The model under review builds one solid part; all positions refer to its coordinate system, in mm. Coordinates: 2 decimals unless noted, no trailing zeros. Order: outer loops, then holes, each group sorted by start corner. A loop starts at its lowest first (then second) coordinate and runs counter-clockwise, first axis right, second up. Notation, with made-up numbers: (17, 54.25) - (67, 54.25) arc R20 ccw to (67, 77.25) - close; hole circle Ø7 at (64.5, 70). An arc over 180 degrees is marked (long way). Answer in a Markdown table with one row per item.
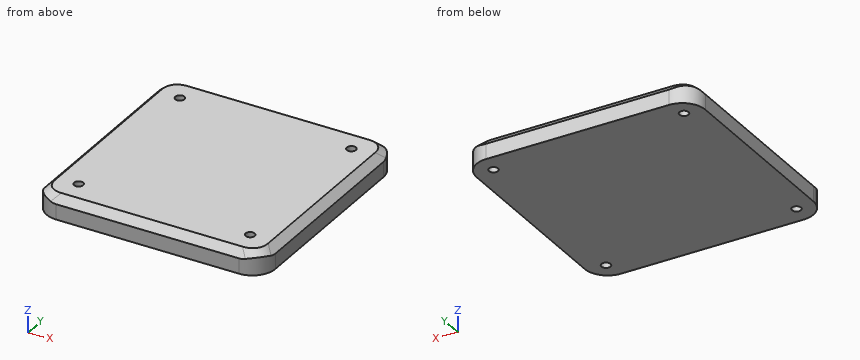
```python
from build123d import *

# Parameters (mm, degrees)
F0_W     = 300
F0_H     = 300
F0_R     = 6
F1_DEPTH = 30
F2_DEPTH = 10
F3_DEPTH = 20
F4_SIZE2 = 10
F4_SIZE  = 10
F5_F1_R  = 30
F5_F2_R  = 30
F5_F3_R  = 30
F5_F4_R  = 30
F5_F5_R  = 30
F5_F6_R  = 30
F5_F7_R  = 30
F5_F8_R  = 30


with BuildPart() as f1:
    # F0 (on Top) → F1 (new body)
    with BuildSketch(Plane.XY):
        Rectangle(F0_W, F0_H)
        with Locations((-125, -125)):
            Circle(F0_R, mode=Mode.SUBTRACT)
        with Locations((-112.5, -112.5)):
            Circle(F0_R, mode=Mode.SUBTRACT)
        with Locations((125, -125)):
            Circle(F0_R, mode=Mode.SUBTRACT)
        with Locations((112.5, -112.5)):
            Circle(F0_R, mode=Mode.SUBTRACT)
        with Locations((-125, 125)):
            Circle(F0_R, mode=Mode.SUBTRACT)
        with Locations((-112.5, 112.5)):
            Circle(F0_R, mode=Mode.SUBTRACT)
        with Locations((112.5, 112.5)):
            Circle(F0_R, mode=Mode.SUBTRACT)
        with Locations((125, 125)):
            Circle(F0_R, mode=Mode.SUBTRACT)
        with Locations((-125, -125)):
            Circle(F0_R)
        with Locations((-125, 125)):
            Circle(F0_R)
        with Locations((125, 125)):
            Circle(F0_R)
        with Locations((125, -125)):
            Circle(F0_R)
    extrude(amount=F1_DEPTH)

    # F0 (on Top) → F2 (cut)
    with BuildSketch(Plane.XY):
        with Locations((-125, -125)):
            Circle(F0_R)
        with Locations((-125, 125)):
            Circle(F0_R)
        with Locations((125, 125)):
            Circle(F0_R)
        with Locations((125, -125)):
            Circle(F0_R)
    extrude(amount=F2_DEPTH, mode=Mode.SUBTRACT)

    # F0 (on Top) → F3 (join)
    with BuildSketch(Plane.XY):
        with Locations((-112.5, 112.5)):
            Circle(F0_R)
        with Locations((-112.5, -112.5)):
            Circle(F0_R)
        with Locations((112.5, 112.5)):
            Circle(F0_R)
        with Locations((112.5, -112.5)):
            Circle(F0_R)
    extrude(amount=F3_DEPTH)

    # F4
    f4_edges = [f1.edges().sort_by_distance(p)[0] for p in [
        (0, -150, 30),
        (-150, 0, 30),
        (150, 0, 30),
        (0, 150, 30),
    ]]
    chamfer(f4_edges, length=F4_SIZE, length2=F4_SIZE2)

    # F5: fillet of radius 30 on 8 edges, made by hand

    # F5_f1
    f5_f1_edges = [f1.edges().sort_by_distance(p)[0] for p in [
        (-150, -150, 10),
    ]]
    fillet(f5_f1_edges, radius=F5_F1_R)

    # F5_f2
    f5_f2_edges = [f1.edges().sort_by_distance(p)[0] for p in [
        (150, -150, 10),
    ]]
    fillet(f5_f2_edges, radius=F5_F2_R)

    # F5_f3
    f5_f3_edges = [f1.edges().sort_by_distance(p)[0] for p in [
        (-150, 150, 10),
    ]]
    fillet(f5_f3_edges, radius=F5_F3_R)

    # F5_f4
    f5_f4_edges = [f1.edges().sort_by_distance(p)[0] for p in [
        (-140.6066017178, -140.6066017178, 29.3933982822),
    ]]
    fillet(f5_f4_edges, radius=F5_F4_R)

    # F5_f5
    f5_f5_edges = [f1.edges().sort_by_distance(p)[0] for p in [
        (140.6066017178, -140.6066017178, 29.3933982822),
    ]]
    fillet(f5_f5_edges, radius=F5_F5_R)

    # F5_f6
    f5_f6_edges = [f1.edges().sort_by_distance(p)[0] for p in [
        (150, 150, 10),
    ]]
    fillet(f5_f6_edges, radius=F5_F6_R)

    # F5_f7
    f5_f7_edges = [f1.edges().sort_by_distance(p)[0] for p in [
        (-140.6066017178, 140.6066017178, 29.3933982822),
    ]]
    fillet(f5_f7_edges, radius=F5_F7_R)

    # F5_f8
    f5_f8_edges = [f1.edges().sort_by_distance(p)[0] for p in [
        (140.6066017178, 140.6066017178, 29.3933982822),
    ]]
    fillet(f5_f8_edges, radius=F5_F8_R)


solid = f1.part
```
Item 1: We need section A-A, the plane y = -112.5. Write out the cut boundary in (x, z).
Check values:
| item | result |
|---|---|
| outline | (-150, 0) - (150, 0) - (150, 20) - (140, 30) - (118.5, 30) - (118.5, 20) - (106.5, 20) - (106.5, 30) - (-106.5, 30) - (-106.5, 20) - (-118.5, 20) - (-118.5, 30) - (-140, 30) - (-150, 20) - close |
Item 2: To check wall thickness, follow line 1 (Y direction, x = 125, z = 4.75); line 2 (Y direction, x = -112.5, z = 23.75); line 3 (X direction, y = 120, z = 1). State the ranges of each line that lie inside material, in increasing order. Write a range as from..to.
Check values:
| item | result |
|---|---|
| line 1 | -149.58..-131, -119..119, 131..149.58 |
| line 2 | -146.25..-118.5, -106.5..106.5, 118.5..146.25 |
| line 3 | -150..-128.32, -121.68..121.68, 128.32..150 |
Item 3: Clearance check with flat-ended pins moving along their axes: pin 1 Ø6 at (x, y) = (114.5, -112) entering from +Z; pin 2 Ø8 at (y, z) = (54.5, 27) entering from -X; pin 3 Ø3 at (x, z) = (11.5, 22.5) entering from -Y. State where each tip first meets the part, or that it passes through.
Check values:
| item | result |
|---|---|
| pin 1 | z = 20 |
| pin 2 | x = -147 |
| pin 3 | y = -149 |
